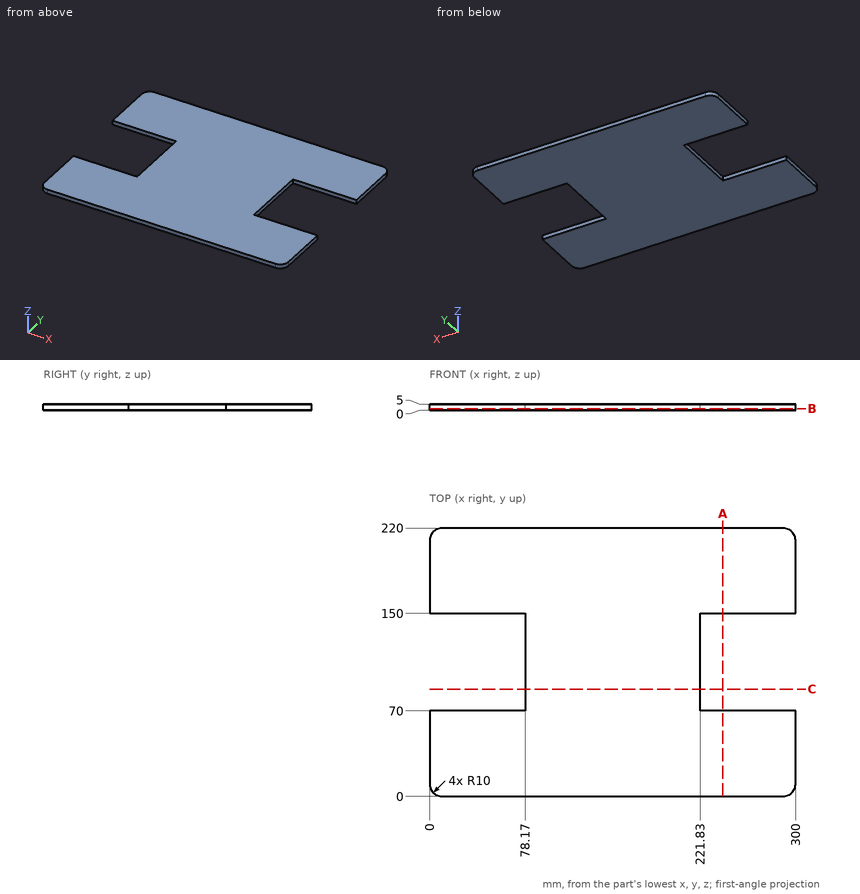
The figure shows three views and two pictorial views of one solid part (mm, origin at its lowest corner). Answer the questions. Give positions to 0.01 mm unless a question says otherwise; leave off trailing zeros. Write each loop counter-clockwise with the first axis right and the second up, starting at its lowest first coordinate (ties: lowest second). Pieces come first, ordered by that corner, then holes. Notation, with made-up numbers: (14.25, 41.5) -> (50.25, 41.5) arc R17 ccw to (50.25, 68.5) -> close; hole circle Ø9 at (-6.75, 62). An arc over 180 degrees is marked (long way). Answer as a JSON object with one key per item and string values.
1) Section B-B on z = 1.2 is taken. Write down the section's boundary in (x, y).
Findings below:
{"outline": "(0, 10) arc R10 ccw to (10, 0) -> (290, 0) arc R10 ccw to (300, 10) -> (300, 70) -> (221.83, 70) -> (221.83, 150) -> (300, 150) -> (300, 210) arc R10 ccw to (290, 220) -> (10, 220) arc R10 ccw to (0, 210) -> (0, 150) -> (78.17, 150) -> (78.17, 70) -> (0, 70) -> close"}
2) Straight lines are drawn through the part: probe 1 along Y at (x, z) = (64, 3.4); probe 2 along X at (y, z) = (120.5, 3.8); probe 3 along X at (y, z) = (211, 0.45). For each, find the intervals that lie inside material, in ascending order. Write a range as from..to.
Findings below:
{"probe 1": "y = 0..70, 150..220", "probe 2": "x = 78.17..221.83", "probe 3": "x = 0.05..299.95"}
3) Section A-A on x = 240.5 is taken. Write down the section's boundary in (y, z).
Findings below:
{"outline": "(0, 0) -> (70, 0) -> (70, 5) -> (0, 5) -> close; (150, 0) -> (220, 0) -> (220, 5) -> (150, 5) -> close"}
4) Section C-C on y = 88 is taken. Write down the section's boundary in (x, z).
Findings below:
{"outline": "(78.17, 0) -> (221.83, 0) -> (221.83, 5) -> (78.17, 5) -> close"}
